from build123d import *

# Parameters (mm, degrees)
BOSS_EXTRUDE1_DEPTH = 250
LPATTERN1_COUNT     = 10
LPATTERN1_PITCH     = 25


with BuildPart() as part:
    # Sketch1 → Boss-Extrude1 (new body)
    with BuildSketch(Plane.XY):
        Polygon((-6, 0), (6, 0), (6, 4.25), (5.25, 5), (4.5, 5), (4.5, 6), (5.25, 6), (6, 6.75), (6, 8), (-6, 8), (-6, 6.75), (-5.25, 6), (-4.5, 6), (-4.5, 5), (-5.25, 5), (-6, 4.25), align=None)
    extrude(amount=BOSS_EXTRUDE1_DEPTH)

    # Sketch2 → Cut-Revolve3 (revolve, cut)
    with BuildSketch(Plane(origin=(0, 0, 0), x_dir=(0, 0, -1), z_dir=(1, 0, 0))):
        Polygon((-10.75, 0), (-10.75, 3.5), (-9.5, 3.5), (-9.5, 8), (-12.5, 8), (-12.5, 0), align=None)
    cut_revolve3 = revolve(axis=Axis((0, 0, 12.5), (0, 1, 0)), mode=Mode.SUBTRACT)

    # LPattern1: Cut-Revolve3 ×10
    with Locations(*[(0, 0, i * LPATTERN1_PITCH) for i in range(1, LPATTERN1_COUNT)]):
        add(cut_revolve3, mode=Mode.SUBTRACT)


solid = part.part
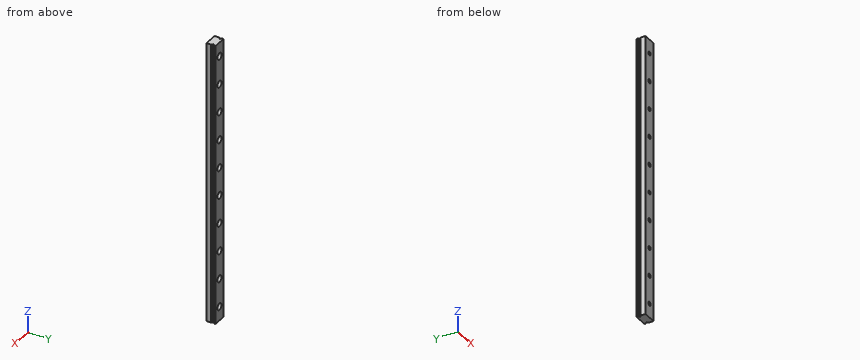
Source: CAD feature listing. Evaluate the final solid. Frame: model axes, mm. Coordinates: 2 decimals unless noted, no trailing zeros. Loops run counter-clockwise (first coordinate to the right, second up) from the corner with the lowest first, then second, coordinate; pieces in that order, holes last. Notation, with made-up numbers: (85, -40) -> (117, -40) arc R35 ccw to (117, -2) -> close; hole circle Ø5 at (40.5, 51). An arc over 180 degrees is marked (long way). Answer in a Markdown table with one row per item. Add a question column.
Q1. Section A-A on z = 54. Return the cut outline in (x, y), and give its area (3 significant figures).
Q2. Contact query for flat-ended pins moving along their axis: pin 1 Ø5 at (x, z) = (0, 187.5) entering from +Y; pin 2 Ø1 at (y, z) = (5, 167.5) entering from +X. Output: stop coordinate, or through.
Q3. Ray query, line 1 along X through (y, z) = (0.8, 112.5); line 2 along X through (y, z) = (5.7, 237.5); line 3 along Y through (x, z) = (0, 239.5). Return the intervals inside material, ascending.
Computed values:
| question | item | result |
|---|---|---|
| 1 | outline | (-6, 0) -> (6, 0) -> (6, 4.25) -> (5.25, 5) -> (4.5, 5) -> (4.5, 6) -> (5.25, 6) -> (6, 6.75) -> (6, 8) -> (-6, 8) -> (-6, 6.75) -> (-5.25, 6) -> (-4.5, 6) -> (-4.5, 5) -> (-5.25, 5) -> (-6, 4.25) -> close |
| 1 | area | 91.9 mm^2 |
| 2 | pin 1 | stops at y = 3.5 |
| 2 | pin 2 | stops at x = 5.75 |
| 3 | line 1 | x = -6 to -1.75, 1.75 to 6 |
| 3 | line 2 | x = -4.5 to -3, 3 to 4.5 |
| 3 | line 3 | y = 0 to 3.5 |
